from build123d import *

# Parameters (mm, degrees)
SKETCH1_W           = 80
SKETCH1_H           = 25
BOSS_EXTRUDE1_DEPTH = 4
SKETCH2_W           = 80
SKETCH2_H           = 4
BOSS_EXTRUDE2_DEPTH = 20
SKETCH3_R           = 3.042773103
BOSS_EXTRUDE3_DEPTH = 80
SKETCH4_R           = 2
CUT_EXTRUDE1_DEPTH  = 80
SKETCH5_R           = 2
CUT_EXTRUDE2_DEPTH  = 80


with BuildPart() as part:
    # Sketch1 → Boss-Extrude1 (new body)
    with BuildSketch(Plane(origin=(0, 0, 0), x_dir=(1, 0, 0), z_dir=(0, 1, 0))):
        Rectangle(SKETCH1_W, SKETCH1_H)
    extrude(amount=BOSS_EXTRUDE1_DEPTH)

    # Sketch2 → Boss-Extrude2 (add)
    with BuildSketch(Plane(origin=(0, 4, 0), x_dir=(1, 0, 0), z_dir=(0, 1, 0))):
        with Locations((0, 10.5)):
            Rectangle(SKETCH2_W, SKETCH2_H)
    extrude(amount=BOSS_EXTRUDE2_DEPTH)

    # Sketch3 → Boss-Extrude3 (add)
    with BuildSketch(Plane.ZY.offset(40)):
        with Locations((-10.673404756, 2.028198383)):
            Circle(SKETCH3_R)
    extrude(amount=-BOSS_EXTRUDE3_DEPTH)

    # Sketch4 → Cut-Extrude1 (cut)
    with BuildSketch(Plane(origin=(0, 0, -12.5), x_dir=(-1, 0, 0), z_dir=(0, 0, -1))):
        with Locations((30, 14.461718051)):
            Circle(SKETCH4_R)
        with Locations((-10, 14)):
            Circle(SKETCH4_R)
        with Locations((10, 19)):
            Circle(SKETCH4_R)
        with Locations((-30, 19)):
            Circle(SKETCH4_R)
    extrude(amount=-CUT_EXTRUDE1_DEPTH, mode=Mode.SUBTRACT)

    # Sketch5 → Cut-Extrude2 (cut)
    with BuildSketch(Plane.XZ):
        with Locations(Location((-30, 2.5, 0), (0, 0, 270))):
            Circle(SKETCH5_R)
        with Locations(Location((-10, 7.5, 0), (0, 0, 270))):
            Circle(SKETCH5_R)
        with Locations(Location((10, 2.5, 0), (0, 0, 270))):
            Circle(SKETCH5_R)
        with Locations(Location((30, 7.5, 0), (0, 0, 270))):
            Circle(SKETCH5_R)
    extrude(amount=-CUT_EXTRUDE2_DEPTH, mode=Mode.SUBTRACT)


solid = part.part
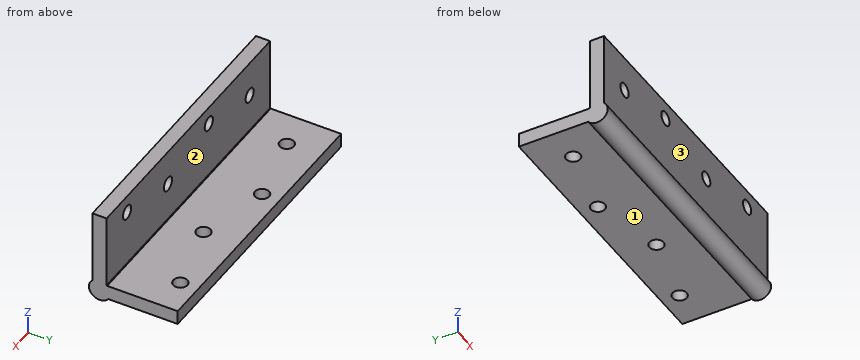
Work out the finished part from the listing and answer in its coordinate system (mm). Face numbers are marked on the shaded views. A direction names the side the tool comes from. Coordinates: 2 decimals unless noted, no trailing zeros. Loops run counter-clockwise (first coordinate to the right, second up) from the corner with the lowest first, then second, coordinate; pieces in that order, holes last. Notation, with made-up numbers: M 68,3 L 98,3 A12 cw 98,7 Z; hole C 77,-12.75 d9. An arc over 180 degrees is marked long. Answer in a Markdown table with one row per item. Add a question column.
1. Find section A-A, the plane z = 2.5. Write down the section's boundary in (x, y).
2. Find section C-C, the plane y = 18. Write down the section's boundary in (x, z).
3. Find section B-B, the plane x = 10. Write down the section's boundary in (y, z).
4. Flat-ended cylindrical pins translate along their axes: P1, Ø4.5, axis at x = -30, z = 2.5, coming from the +Y side; P2, Ø10.5, axis at x = -10.5, z = -2, coming from the -Y side; P3, Ø6.5, axis at x = -10, y = 19, coming from the +Z side. Find the tip coordinate at first contact, or state that the pin passes through.
5. A tool of negligible diameter and unlimited length cuts with its end or side. For the marked faces 1, 2 and 3, from which of +Z, -Z, +X, -X, +Y, -Y can it reach the whole face along a straight path? Write none if from no direction.
6. Find section D-D, the plane z = -10.25. Write down the section's boundary in (x, y).
7. Consider L1, parallel to X at y = 2.3, z = 2.5; L2, parallel to Y at x = 30, z = -10.8; L3, parallel to Y at x = -30, z = -10.7. Determine where each line is inside the solid, lowest interval first.
Reported:
| question | item | result |
|---|---|---|
| 1 | outline | M -40,0 L -32,0 L -32,4 L -40,4 Z; M -28,0 L 8,0 L 8,4 L -28,4 Z; M 12,0 L 40,0 L 40,4 L 12,4 Z |
| 2 | outline | M -40,-12.5 L -11.73,-12.5 L -11.73,-8.5 L -40,-8.5 Z; M -8.27,-12.5 L 28.27,-12.5 L 28.27,-8.5 L -8.27,-8.5 Z; M 31.73,-12.5 L 40,-12.5 L 40,-8.5 L 31.73,-8.5 Z |
| 3 | outline | M 0,-8.41 A3.04 ccw long 4.46,-12.5 L 12,-12.5 L 12,-8.5 L 4.16,-8.5 A3.04 ccw 4,-8.36 L 4,0.5 L 0,0.5 Z; M 0,4.5 L 4,4.5 L 4,12.5 L 0,12.5 Z; M 16,-12.5 L 24,-12.5 L 24,-8.5 L 16,-8.5 Z |
| 4 | P1 | stops at y = 4 |
| 4 | P2 | stops at y = 0 |
| 4 | P3 | stops at z = -8.5 |
| 5 | face 1 | -Z, +X, -X, +Y |
| 5 | face 2 | +Z, +X, -X, +Y |
| 5 | face 3 | +Z, +X, -X, -Y |
| 6 | outline | M -40,-0.98 L 40,-0.98 L 40,24 L -40,24 Z; hole C -30,14.46 d4; hole C -10,19 d4; hole C 10,14 d4; hole C 30,19 d4 |
| 7 | L1 | x = -40 to -32, -28 to 8, 12 to 40 |
| 7 | L2 | y = -1.01 to 17, 21 to 24 |
| 7 | L3 | y = -1.01 to 12.46, 16.46 to 24 |
